Work out the finished part from the listing and answer in its coordinate system (mm). A direction names the side the tool comes from. Round coordinates to 2 decimals unless told otherwise and drop trailing zeros. Order: outer loops, then holes, each group sorted by start corner. A loop starts at its lowest first (then second) coordinate and runs counter-clockwise, first axis right, second up. Notation, with made-up numbers: M 37,19 L 81,19 A32 cw 81,48 Z; hole C 55,-20.75 d2. An arc over 180 degrees is marked long. Answer as a JSON object with one key per item and string values. Group by question number.
from build123d import *

# Parameters (mm, degrees)
SKETCH1_W           = 72
SKETCH1_H           = 100
SKETCH1_R           = 1.5
BOSS_EXTRUDE1_DEPTH = 3
SKETCH3_W           = 13
SKETCH3_H           = 10
BOSS_EXTRUDE3_DEPTH = 11
CUT_EXTRUDE1_DEPTH  = 15
SKETCH6_R           = 3.1
CUT_EXTRUDE2_DEPTH  = 10.913949805
FILLET1_R           = 4
SKETCH7_R           = 1.5
CUT_EXTRUDE3_DEPTH  = 8.537088113


with BuildPart() as part:
    # Sketch1 → Boss-Extrude1 (new body)
    with BuildSketch(Plane.XZ):
        with Locations((39, 0)):
            Rectangle(SKETCH1_W, SKETCH1_H)
        with Locations((7, -45.5)):
            Circle(SKETCH1_R, mode=Mode.SUBTRACT)
        with BuildLine():
            Line((62, 37), (62, -37))
            ThreePointArc((62, -37), (60.535533906, -40.535533906), (57, -42))
            Line((57, -42), (16, -42))
            ThreePointArc((16, -42), (12.464466094, -40.535533906), (11, -37))
            Line((11, -37), (11, 37))
            ThreePointArc((11, 37), (12.464466094, 40.535533906), (16, 42))
            Line((16, 42), (57, 42))
            ThreePointArc((57, 42), (60.535533906, 40.535533906), (62, 37))
        make_face(mode=Mode.SUBTRACT)
        with Locations((7, 45.5)):
            Circle(SKETCH1_R, mode=Mode.SUBTRACT)
    extrude(amount=BOSS_EXTRUDE1_DEPTH)

    # Sketch3 → Boss-Extrude3 (add)
    with BuildSketch(Plane.XZ.offset(3)):
        with Locations((68.5, -41.227292579)):
            Rectangle(SKETCH3_W, SKETCH3_H)
    boss_extrude3 = extrude(amount=BOSS_EXTRUDE3_DEPTH)

    # Sketch4 → Cut-Extrude1 (cut)
    with BuildSketch(Plane(origin=(0, 0, -46.227292579), x_dir=(-1, 0, 0), z_dir=(0, 0, -1))):
        Polygon((-62, -14), (-62, -3), (-70.723130932, -9.108002035), (-67.29771708, -14), align=None)
        Polygon((-67.29771708, -14), (-70.723130932, -9.108002035), (-75, -3), (-75, -14), align=None)
    cut_extrude1 = extrude(amount=-CUT_EXTRUDE1_DEPTH, mode=Mode.SUBTRACT)

    # Sketch6 → Cut-Extrude2 (cut, through all)
    with BuildSketch(Plane(origin=(18.987836626, 27.117441029, 0), x_dir=(0.819152044, -0.573576436, 0), z_dir=(-0.573576436, -0.819152044, 0))):
        with Locations((55.50325926, -41.227292579)):
            Circle(SKETCH6_R)
    cut_extrude2 = extrude(amount=-CUT_EXTRUDE2_DEPTH, mode=Mode.SUBTRACT)

    # Mirror1: Boss-Extrude3, Cut-Extrude1, Cut-Extrude2 across plane
    add(boss_extrude3.mirror(Plane.XY))
    add(cut_extrude1.mirror(Plane.XY), mode=Mode.SUBTRACT)
    add(cut_extrude2.mirror(Plane.XY), mode=Mode.SUBTRACT)

    # Fillet1
    fillet1_edges = [part.edges().sort_by_distance(p)[0] for p in [
        (70.723130932, -9.108002035, 41.227292579),
        (70.723130932, -9.108002035, -41.227292579),
    ]]
    fillet(fillet1_edges, radius=FILLET1_R)

    # Sketch7 → Cut-Extrude3 (cut, through all)
    with BuildSketch(Plane(origin=(0, 0, 0), x_dir=(1, 0, 0), z_dir=(0, 1, 0))):
        with Locations((69, 30)):
            Circle(SKETCH7_R)
        with Locations((69, -30)):
            Circle(SKETCH7_R)
    extrude(amount=-CUT_EXTRUDE3_DEPTH, mode=Mode.SUBTRACT)


solid = part.part
Item 1: Consider L1, parallel to Z at x = 7, y = -0.8; L2, parallel to X at y = -1.9, z = 30; L3, parallel to X at y = -1.5, z = -37.5. Determine where each line is inside the solid, lowest interval first.
Item 2: The mould has two halves that part along X. Classify faces 4 (the flat face through (68, -5, 46.227)), 5 (the cylindrical face through (70.43, -1.48, 29.55)), 6 (the flat face through (67.11, -6.58, 40.19)): +X half, -X half, draft (parallel to the pull), parting line (faces both ways), or undercut.
Item 3: Find section C-C (z = -30). Give the vertices of the cut face in (x, y), and give its area (3 significant figures).
Item 4: Find section D-D (x = 22). Give the vertices of the cut face in (y, z).
Item 5: Each of these flat-tipped pins is pushed along its axis until it touches: pin 1 (1 mm diameter, centred on x = 64.5, y = -5, fed in from +Z); pin 2 (14.5 mm diameter, centred on x = 67.5, z = 9.5, fed in from -Y); pin 3 (1.4 mm diameter, centred on x = 66, y = -4.5, fed in from -Z). Where does it stop, or does it pass through?
Item 6: A tool of negligible diameter and unlimited length cuts with its end or side. For faces 1 (the cylindrical face through (61, -1, -40)), 2 (the flat face through (68, -5, 36.227)), 3 (the flat face through (68, -5, -46.227)), from which of +Z, -Z, +X, -X, +Y, -Y can it reach the whole face along a straight path? Write none if from no direction.
Item 7: Find section A-A (z = 3). Give the vertices of the cut face in (x, y), and give its area (3 significant figures).
Item 8: Find section B-B (x = 7). Give the vertices of the cut face in (y, z), and give its area (3 significant figures).
Responses:
{
 "1": {"L1": "z = -50 to -47, -44 to 44, 47 to 50", "L2": "x = 3 to 11, 62 to 67.5, 70.5 to 75", "L3": "x = 3 to 11.03, 61.97 to 75"},
 "2": {"face 4": "draft", "face 5": "undercut", "face 6": "-X half"},
 "3": {"outline": "M 3,-3 L 11,-3 L 11,0 L 3,0 Z; M 62,-3 L 67.5,-3 L 67.5,0 L 62,0 Z; M 70.5,-3 L 75,-3 L 75,0 L 70.5,0 Z", "area": "54.0 mm^2"},
 "4": {"outline": "M -3,-50 L 0,-50 L 0,-42 L -3,-42 Z; M -3,42 L 0,42 L 0,50 L -3,50 Z"},
 "5": {"pin 1": "stops at z = 46.23", "pin 2": "stops at y = -3", "pin 3": "stops at z = -46.23"},
 "6": {"face 1": "+Y, -Y", "face 2": "+X, -X, -Y", "face 3": "-Z, +X, -X, -Y"},
 "7": {"outline": "M 3,-3 L 11,-3 L 11,0 L 3,0 Z; M 62,-3 L 75,-3 L 75,0 L 62,0 Z", "area": "63.0 mm^2"},
 "8": {"outline": "M -3,-50 L 0,-50 L 0,-47 L -3,-47 Z; M -3,-44 L 0,-44 L 0,44 L -3,44 Z; M -3,47 L 0,47 L 0,50 L -3,50 Z", "area": "282 mm^2"}
}
